```python
from build123d import *

# Parameters (mm, degrees)
SKETCH1_W               = 55
SKETCH1_H               = 22
BOSS_EXTRUDE1_DEPTH     = 10
CUT_EXTRUDE1_DEPTH      = 32.260998065
CUT_EXTRUDE1_DEPTH_BACK = 32.260998065
SKETCH2_R               = 1.8
BOSS_EXTRUDE2_START     = -27.5
BOSS_EXTRUDE2_DEPTH     = 4
BOSS_EXTRUDE3_START     = 23.5
BOSS_EXTRUDE3_DEPTH     = 4
CUT_EXTRUDE2_START      = -23.5
SKETCH4_R               = 3.5
CUT_EXTRUDE2_DEPTH      = 2
CUT_EXTRUDE2_DRAFT      = -30
CUT_EXTRUDE3_START      = 23.5
SKETCH4_2_R             = 3.5
CUT_EXTRUDE3_DEPTH      = 2
CUT_EXTRUDE3_TAPER      = 30
CUT_EXTRUDE4_DEPTH      = 23
BOSS_EXTRUDE4_START     = 27.5
BOSS_EXTRUDE4_DEPTH     = 3
BOSS_EXTRUDE4_TAPER     = 25
BOSS_EXTRUDE5_START     = -27.5
BOSS_EXTRUDE5_DEPTH     = 3
BOSS_EXTRUDE5_DRAFT     = -25
CUT_EXTRUDE5_START      = 30.5
SKETCH7_R               = 3
CUT_EXTRUDE5_DEPTH      = 1
CUT_EXTRUDE6_START      = -29.5
SKETCH7_2_R             = 3
CUT_EXTRUDE6_DEPTH      = 1
CUT_EXTRUDE7_START      = 27.5
CUT_EXTRUDE7_DEPTH      = 1
CUT_EXTRUDE8_START      = -26.5
CUT_EXTRUDE8_DEPTH      = 1
SKETCH9_R               = 7.00121046
BOSS_EXTRUDE6_DEPTH     = 0.3
FILLET1_R               = 0.8


with BuildPart() as part:
    # Sketch1 → Boss-Extrude1 (new body)
    with BuildSketch(Plane.XY):
        Rectangle(SKETCH1_W, SKETCH1_H)
    extrude(amount=BOSS_EXTRUDE1_DEPTH)

    # Sketch2 → Cut-Extrude1 (cut, two sides: drawn at the far end of the back side and taken through both)
    with BuildSketch(Plane(origin=(0, 0, 0), x_dir=(1, 0, 0), z_dir=(0, 1, 0)).offset(-CUT_EXTRUDE1_DEPTH_BACK)):
        with Locations(Location((-17.5, -4, 0), (0, 0, 270))):
            Circle(SKETCH2_R)
        with Locations(Location((17.5, -4, 0), (0, 0, 270))):
            Circle(SKETCH2_R)
    extrude(amount=CUT_EXTRUDE1_DEPTH + CUT_EXTRUDE1_DEPTH_BACK, mode=Mode.SUBTRACT)

    # Sketch3 → Boss-Extrude2 (add)
    with BuildSketch(Plane(origin=(0, 0, 0), x_dir=(0, 0, -1), z_dir=(1, 0, 0)).offset(BOSS_EXTRUDE2_START)):
        with BuildLine():
            Line((-31.151137667, 4.83507467), (-10, 11))
            Line((-10, 11), (-10, -11))
            Line((-10, -11), (-31.167743327, -4.892335032))
            ThreePointArc((-31.167743327, -4.892335032), (-34.999992715, -0.022073975), (-31.151137667, 4.83507467))
        make_face()
    extrude(amount=BOSS_EXTRUDE2_DEPTH)

    # Sketch3<2> → Boss-Extrude3 (add)
    with BuildSketch(Plane(origin=(0, 0, 0), x_dir=(0, 0, -1), z_dir=(1, 0, 0)).offset(BOSS_EXTRUDE3_START)):
        with BuildLine():
            Line((-31.151137667, 4.83507467), (-10, 11))
            Line((-10, 11), (-10, -11))
            Line((-10, -11), (-31.167743327, -4.892335032))
            ThreePointArc((-31.167743327, -4.892335032), (-34.999992715, -0.022073975), (-31.151137667, 4.83507467))
        make_face()
    extrude(amount=BOSS_EXTRUDE3_DEPTH)


with BuildPart() as cut_extrude2_tool:
    # Sketch4 → Cut-Extrude2 (with draft: the straight prism first)
    with BuildSketch(Plane(origin=(0, 0, 0), x_dir=(0, 0, -1), z_dir=(1, 0, 0)).offset(CUT_EXTRUDE2_START)):
        with Locations((-30, 0)):
            Circle(SKETCH4_R)
    extrude(amount=-CUT_EXTRUDE2_DEPTH)
    # Cut-Extrude2: the draft: its side faces are tilted about the plane it starts from
    cut_extrude2_sides = [cut_extrude2_tool.faces().sort_by_distance(p)[0] for p in [
        (-24.5, 0, 33.5),
    ]]
    draft(cut_extrude2_sides, Plane(origin=(0, 0, 0), x_dir=(0, 0, -1), z_dir=(1, 0, 0)).offset(CUT_EXTRUDE2_START), CUT_EXTRUDE2_DRAFT)


with BuildPart() as part_1:
    add(part.part)

    # Cut-Extrude2: cut by cut_extrude2_tool
    add(cut_extrude2_tool.part, mode=Mode.SUBTRACT)

    # Sketch4<2> → Cut-Extrude3 (cut)
    with BuildSketch(Plane(origin=(0, 0, 0), x_dir=(0, 0, -1), z_dir=(1, 0, 0)).offset(CUT_EXTRUDE3_START)):
        with Locations((-30, 0)):
            Circle(SKETCH4_2_R)
    extrude(amount=CUT_EXTRUDE3_DEPTH, taper=CUT_EXTRUDE3_TAPER, mode=Mode.SUBTRACT)

    # Sketch5 → Cut-Extrude4 (cut, symmetric)
    with BuildSketch(Plane(origin=(0, 0, 0), x_dir=(0, 0, -1), z_dir=(1, 0, 0))):
        with BuildLine():
            Line((-20.614301305, 18.586324402), (-20.058086713, -18.355544485))
            ThreePointArc((-20.058086713, -18.355544485), (-8.002266591, 0.301095517), (-20.614301305, 18.586324402))
        make_face()
    extrude(amount=CUT_EXTRUDE4_DEPTH, both=True, mode=Mode.SUBTRACT)

    # Sketch6 → Boss-Extrude4 (add)
    with BuildSketch(Plane(origin=(0, 0, 0), x_dir=(0, 0, -1), z_dir=(1, 0, 0)).offset(BOSS_EXTRUDE4_START)):
        with BuildLine():
            Line((0, -5), (0, 5))
            Line((0, 5), (-5, 5))
            ThreePointArc((-5, 5), (-10, 0), (-5, -5))
            Line((-5, -5), (0, -5))
        make_face()
    extrude(amount=BOSS_EXTRUDE4_DEPTH, taper=BOSS_EXTRUDE4_TAPER)


with BuildPart() as boss_extrude5_tool:
    # Sketch6<2> → Boss-Extrude5 (with draft: the straight prism first)
    with BuildSketch(Plane(origin=(0, 0, 0), x_dir=(0, 0, -1), z_dir=(1, 0, 0)).offset(BOSS_EXTRUDE5_START)):
        with BuildLine():
            Line((0, -5), (0, 5))
            Line((0, 5), (-5, 5))
            ThreePointArc((-5, 5), (-10, 0), (-5, -5))
            Line((-5, -5), (0, -5))
        make_face()
    extrude(amount=-BOSS_EXTRUDE5_DEPTH)
    # Boss-Extrude5: the draft: its side faces are tilted about the plane it starts from
    boss_extrude5_sides = [boss_extrude5_tool.faces().sort_by_distance(p)[0] for p in [
        (-29, -5, 2.5),
        (-29, 0, 0),
        (-29, 5, 2.5),
        (-29, 0, 10),
    ]]
    draft(boss_extrude5_sides, Plane(origin=(0, 0, 0), x_dir=(0, 0, -1), z_dir=(1, 0, 0)).offset(BOSS_EXTRUDE5_START), BOSS_EXTRUDE5_DRAFT)


with BuildPart() as part_2:
    add(part_1.part)

    # Boss-Extrude5: add boss_extrude5_tool
    add(boss_extrude5_tool.part)

    # Sketch7 → Cut-Extrude5 (cut)
    with BuildSketch(Plane(origin=(0, 0, 0), x_dir=(0, 0, -1), z_dir=(1, 0, 0)).offset(CUT_EXTRUDE5_START)):
        with Locations(Location((-5, 0, 0), (0, 0, 270))):
            Circle(SKETCH7_R)
    extrude(amount=-CUT_EXTRUDE5_DEPTH, mode=Mode.SUBTRACT)

    # Sketch7<2> → Cut-Extrude6 (cut)
    with BuildSketch(Plane(origin=(0, 0, 0), x_dir=(0, 0, -1), z_dir=(1, 0, 0)).offset(CUT_EXTRUDE6_START)):
        with Locations(Location((-5, 0, 0), (0, 0, 270))):
            Circle(SKETCH7_2_R)
    extrude(amount=-CUT_EXTRUDE6_DEPTH, mode=Mode.SUBTRACT)

    # Sketch8 → Cut-Extrude7 (cut)
    with BuildSketch(Plane(origin=(0, 0, 0), x_dir=(0, 0, -1), z_dir=(1, 0, 0)).offset(CUT_EXTRUDE7_START)):
        with BuildLine():
            Line((-11.878371675, 4.672816565), (-11.878371675, -4.672816565))
            ThreePointArc((-11.878371675, -4.672816565), (-12.676601149, -6.271487138), (-14.434119277, -6.594051741))
            Line((-14.434119277, -6.594051741), (-21.789358175, -4.466432788))
            ThreePointArc((-21.789358175, -4.466432788), (-22.985578278, -3.509878473), (-23.154296174, -1.987553618))
            ThreePointArc((-23.154296174, -1.987553618), (-22.871603949, 0), (-23.154296174, 1.987553618))
            ThreePointArc((-23.154296174, 1.987553618), (-22.985578278, 3.509878473), (-21.789358175, 4.466432788))
            Line((-21.789358175, 4.466432788), (-14.434119277, 6.594051741))
            ThreePointArc((-14.434119277, 6.594051741), (-12.676601149, 6.271487138), (-11.878371675, 4.672816565))
        make_face()
    extrude(amount=-CUT_EXTRUDE7_DEPTH, mode=Mode.SUBTRACT)

    # Sketch8<2> → Cut-Extrude8 (cut)
    with BuildSketch(Plane(origin=(0, 0, 0), x_dir=(0, 0, -1), z_dir=(1, 0, 0)).offset(CUT_EXTRUDE8_START)):
        with BuildLine():
            Line((-11.878371675, 4.672816565), (-11.878371675, -4.672816565))
            ThreePointArc((-11.878371675, -4.672816565), (-12.676601149, -6.271487138), (-14.434119277, -6.594051741))
            Line((-14.434119277, -6.594051741), (-21.789358175, -4.466432788))
            ThreePointArc((-21.789358175, -4.466432788), (-22.985578278, -3.509878473), (-23.154296174, -1.987553618))
            ThreePointArc((-23.154296174, -1.987553618), (-22.871603949, 0), (-23.154296174, 1.987553618))
            ThreePointArc((-23.154296174, 1.987553618), (-22.985578278, 3.509878473), (-21.789358175, 4.466432788))
            Line((-21.789358175, 4.466432788), (-14.434119277, 6.594051741))
            ThreePointArc((-14.434119277, 6.594051741), (-12.676601149, 6.271487138), (-11.878371675, 4.672816565))
        make_face()
    extrude(amount=-CUT_EXTRUDE8_DEPTH, mode=Mode.SUBTRACT)

    # Sketch9 → Boss-Extrude6 (add)
    with BuildSketch(Plane.XY):
        with Locations((27.5, 11)):
            Circle(SKETCH9_R)
        with Locations((-27.5, 11)):
            Circle(SKETCH9_R)
        with Locations((-27.5, -11)):
            Circle(SKETCH9_R)
        with Locations((27.5, -11)):
            Circle(SKETCH9_R)
    extrude(amount=BOSS_EXTRUDE6_DEPTH)

    # Fillet1
    fillet1_edges = [part_2.edges().sort_by_distance(p)[0] for p in [
        (26.5, 0, 22.871603949),
        (26.5, 5.530242265, 18.111738726),
        (26.5, 0, 11.878371675),
        (26.5, -5.530242265, 18.111738726),
        (26.5, -3.509878473, 22.985578278),
        (26.5, 3.509878473, 22.985578278),
        (26.5, 6.271487138, 12.676601149),
        (26.5, -6.271487138, 12.676601149),
        (-26.5, 0, 22.871603949),
        (-26.5, -3.509878473, 22.985578278),
        (-26.5, -5.530242265, 18.111738726),
        (-26.5, -6.271487138, 12.676601149),
        (-26.5, 0, 11.878371675),
        (-26.5, 6.271487138, 12.676601149),
        (-26.5, 5.530242265, 18.111738726),
        (-26.5, 3.509878473, 22.985578278),
        (29.5, 3, 5),
        (-29.5, 3, 5),
    ]]
    fillet(fillet1_edges, radius=FILLET1_R)


solid = part_2.part
```
CAD build for the part. Positions are in the model's coordinates, mm. A direction names the side the tool comes from. Coordinates: 2 decimals unless noted, no trailing zeros. Order: outer loops, then holes, each group sorted by start corner. A loop starts at its lowest first (then second) coordinate and runs counter-clockwise, first axis right, second up. Notation, with made-up numbers: (85.25, -29.5) - (111.25, -29.5) arc R10 ccw to (111.25, -24.5) - close; hole circle Ø4 at (-33.5, 29). An arc over 180 degrees is marked (long way). Use a Markdown table: item, result. Add a question column.
(1) Which spindle directions (+Z, -Z, +X, -X, +Y, -Y) get a long thin tool onto all of the face, cutting with end or side? Do faces 1 (the face through (0, 9, 10)), 2 (the face through (29.5, 0, 5)), 3 (the face through (-29.5, 0, 5)), 4 (the face through (0, 0, 8)), 5 (the face through (25.5, 0, 30)). Say none if no direction does.
(2) Saw through at A-A (x = 17.5). Give the cut face in (y, z), then the cut area to 3 significant figures.
(3) Drill centre lines: line 1 along X through (y, z) = (2, 4); line 2 along X through (y, z) = (5.75, 4); line 3 along X through (y, z) = (-2.5, 21). Where is each one in solid material? Low to high. Write a range as [from, to].
(4) Saw through at D-D (x = -9.5). Give the cut face in (y, z).
(5) Saw through at C-C (z = 30). Give the cut face in (x, y), then the cut area to 3 significant figures.
(6) Pull direction Y, two halves, no side cores. Call faces 6 (the face through (-27.5, 3, 10)), 7 (the face through (-29.646, 0.088, 8.998)), 8 (the face through (-25.37, 0.11, 32.42)): +Y half, -Y half, draft (parallel to the pull), parting line (faces both ways), or undercut.
(7) Flat gauge pins, fed straight in: pin 1 (10.5 mm diameter, centred on y = 2.5, z = 17.5, fed in from -X); pin 2 (1 mm diameter, centred on y = -13, z = 11.5, fed in from +X); pin 3 (12 mm diameter, centred on x = 25.5, z = 19.5, fed in from +Y); pin 4 (5 mm diameter, centred on x = -10.5, z = 6.5, fed in from -Y). Where does each tip first touch, or does it go through?
(8) Saw through at B-B (y = 16). Give the cut face in (x, z), then the cut area to 3 significant figures.
Solved:
| question | item | result |
|---|---|---|
| 1 | face 1 | +Z, +Y, -Y |
| 1 | face 2 | +X |
| 1 | face 3 | -X |
| 1 | face 4 | +Z |
| 1 | face 5 | none |
| 2 | outline | (-11, 0) - (11, 0) - (11, 2.2) - (-11, 2.2) - close; (-11, 5.8) - (11, 5.8) - (11, 10) - (8.72, 10) arc R20 cw to (-8.72, 10) - (-11, 10) - close |
| 2 | area | 117 mm² |
| 3 | line 1 | x = [-29.5, -19.3], [-15.7, 15.7], [19.3, 29.5] |
| 3 | line 2 | x = [-27.5, -19.3], [-15.7, 15.7], [19.3, 27.5] |
| 3 | line 3 | x = [-26.5, -23.5], [23.5, 26.5] |
| 4 | outline | (-11, 0) - (11, 0) - (11, 10) - (8.72, 10) arc R20 cw to (-8.72, 10) - (-11, 10) - close |
| 5 | outline | (-27.5, -5.23) - (-23.5, -5.23) - (-23.5, -3.5) - (-25.5, -2.35) - (-25.5, 2.35) - (-23.5, 3.5) - (-23.5, 5.17) - (-27.5, 5.17) - close; (23.5, -5.23) - (27.5, -5.23) - (27.5, 5.17) - (23.5, 5.17) - (23.5, 3.5) - (25.5, 2.35) - (25.5, -2.35) - (23.5, -3.5) - close |
| 5 | area | 59.8 mm² |
| 6 | face 6 | draft |
| 6 | face 7 | parting line |
| 6 | face 8 | undercut |
| 7 | pin 1 | stops at x = -27.5 |
| 7 | pin 2 | passes through |
| 7 | pin 3 | stops at y = 9.98 |
| 7 | pin 4 | stops at y = -11 |
| 8 | outline | (-32.4, 0) - (-22.6, 0) - (-22.6, 0.3) - (-32.4, 0.3) - close; (22.6, 0) - (32.4, 0) - (32.4, 0.3) - (22.6, 0.3) - close |
| 8 | area | 5.88 mm² |
